Check sheet for the modelled part. Datum: model origin and axes. Units: mm. A direction names the side the tool comes from. Coordinates: 2 decimals unless noted, no trailing zeros. Write each loop counter-clockwise with the first axis right and the second up, starting at its lowest first coordinate (ties: lowest second). Pieces come first, ordered by that corner, then holes. Notation, with made-up numbers: (40, -28.5) - (87, -28.5) arc R34 cw to (87, 3.5) - close; hole circle Ø11 at (47, 31). An arc over 180 degrees is marked (long way). Answer as CSV lines item,"result". Start each with the question number.
from build123d import *

# Parameters (mm, degrees)
F0_R          = 37.465
F0_R_2        = 34.28492
F1_DEPTH      = 33.02
F1_DEPTH_BACK = 33.02
F2_SIZE       = 3.175
F3_R          = 76.2
F4_DEPTH      = 1.5875
F4_DEPTH_BACK = 1.5875
F5_R          = 12.7


with BuildPart() as f1:
    # F0 (on Top) → F1 (new body, two sides)
    with BuildSketch(Plane.XY) as f1_sk:
        Circle(F0_R)
        Circle(F0_R_2, mode=Mode.SUBTRACT)
    extrude(amount=F1_DEPTH)
    extrude(f1_sk.sketch, amount=-F1_DEPTH_BACK)

    # F2
    f2_edges = [f1.edges().sort_by_distance(p)[0] for p in [
        (-37.465, 0, 33.02),
    ]]
    chamfer(f2_edges, length=F2_SIZE)

    # F3 (on Top) → F4 (join, two sides)
    with BuildSketch(Plane.XY) as f4_sk:
        Circle(F3_R)
        with BuildLine():
            ThreePointArc((15.7090324336, -5.08), (-16.51, 0), (15.7090324336, 5.08))
            Line((15.7090324336, 5.08), (27.08475078, 5.08))
            Line((27.08475078, 5.08), (27.08475078, -5.08))
            Line((27.08475078, -5.08), (15.7090324336, -5.08))
        make_face(mode=Mode.SUBTRACT)
    extrude(amount=F4_DEPTH)
    extrude(f4_sk.sketch, amount=-F4_DEPTH_BACK)

    # F5
    f5_edges = [f1.edges().sort_by_distance(p)[0] for p in [
        (-37.465, 0, -1.5875),
    ]]
    fillet(f5_edges, radius=F5_R)


solid = f1.part
(1) Cross-section at C-C on z = 11.5. Record the boundary of the cut face in (x, y) (3 decimals).
(2) Release check for a two-part mould opening along X. For faces 4 (the face through (-7.43, -33.47, -17.08)), 5 (the face through (16, 35, 1.588)), 6 (the face through (-8, -15, -1.588)), 7 (the face through (-29.73, -22.8, 15.91)) record: pulls with the +X half, pulls with the -X half, needs draft (parallel to the pull), parting line crosses it, or undercut.
(3) Tool access check on faces 1 (the face through (-29.73, -22.8, -23.52)), 2 (the face through (-8, -15, 1.588)), 3 (the face through (-60.47, -46.367, 0.022)). Record the directions out of +Z, -Z, +X, -X, +Y, -Y that give a thin tool (end or side, any length) a straight path to the whole face; none if there is none.
(4) Material ranges on probe 1 along Y at (x, z) = (0, 22) (3 decimals); probe 2 along X at (y, z) = (-0.5, 9.5); probe 3 along Y at (x, z) = (0, 0.55), recorded low to high. Write a range as from..to.
(5) Cross-section at D-D on y = 64. Record the boundary of the cut face in (x, z).
(6) Go/stop test with flat-tipped pins: P1, Ø2.5, axis at x = 20.5, z = 0.5, coming from the +Y side; P2, Ø8, axis at y = -48, z = -9.5, coming from the -X side; P3, Ø1.5, axis at x = -13.5, z = -23, coming from the -Y side; P4, Ø12, axis at y = 39, z = 2.5, coming from the +X side. Record where each tip stops, or that it passes through.
Checked values:
1,outline,"circle Ø74.93 at (0, 0); hole circle Ø68.57 at (0, 0)"
2,face 4,"undercut"
2,face 5,"needs draft"
2,face 6,"undercut"
2,face 7,"parting line crosses it"
3,face 1,"-Z"
3,face 2,"+Z"
3,face 3,"+Z, -Z"
4,probe 1,"-37.465..-34.285, 34.285..37.465"
4,probe 2,"-37.46..-34.28, 34.28..37.46"
4,probe 3,"-76.2..-16.51, 16.51..76.2"
5,outline,"(-41.36, -1.59) - (41.36, -1.59) - (41.36, 1.59) - (-41.36, 1.59) - close"
6,P1,"y = 73.73"
6,P2,"through"
6,P3,"y = -35.23"
6,P4,"x = 68.65"
